The model under review builds one solid part; all positions refer to its coordinate system, in mm. A direction names the side the tool comes from. Give positions to 0.01 mm unless a question says otherwise; leave off trailing zeros. Order: outer loops, then holes, each group sorted by start corner. A loop starts at its lowest first (then second) coordinate and runs counter-clockwise, first axis right, second up. Notation, with made-up numbers: (32, -38.75) - (87, -38.75) arc R14 cw to (87, -17.75) - close; hole circle Ø3 at (-4.5, -16). An arc over 180 degrees is marked (long way). Write item = value, one per line. Start each with the question number.
1. We need section C-C, the plane z = -4.75. Give the boundary of the cut face in (x, y).
2. Wall thickness on probe 1 along X at (y, z) = (-35, -5.25); probe 2 along Y at (x, z) = (-35, 8.5); probe 3 along X at (y, z) = (-10, 11.5): over which ranges is each line inside the solid? List them lowest first.
3. Mouldability with a two-part tool opening along Y and no side actions: class faces 4 (the flat face through (-4, -22, 14)), 5 (the cylindrical face through (31.32, -43.472, 18.551)), 6 (the cylindrical face through (-31.836, -1.449, 18.472)), 7 (the cylindrical face through (37.21, -37.03, 5.21)) as pulls with the +Y half, pulls with the -Y half, needs draft (parallel to the pull), parting line crosses it, or undercut.
4. We need section B-B, the plane y = -10. Give the boundary of the cut face in (x, z).
5. Machinability: for faces 1 (the cylindrical face through (4.295, -43.472, 12.246)), 2 (the cylindrical face through (4.295, -1.528, 12.246)), 3 (the cylindrical face through (-10.202, -22.744, 19.404)), which of the approach directions +Z, -Z, +X, -X, +Y, -Y give a long, thin tool a straight path to every point of the face, cutting with its end or side? Answer none if there is none.
6. We need section A-A, the plane x = -35. Give the boundary of the cut face in (y, z).
7. For P1, Ø5, axis at x = -1, y = -10.5, coming from the +Z side; P2, Ø5, axis at x = -35, y = -35, coming from the -Z side, all flat-tipped, find the tip position at first contact; note any pin that passes through.
8. We need section D-D, the plane y = -27.5. Give the boundary of the cut face in (x, z).
from build123d import *

# Parameters (mm, degrees)
F1_DEPTH = 45
F2_R     = 7.62
F3_R     = 5.08
F5_D     = 6


with BuildPart() as f1:
    # F0 (on Front) → F1 (new body)
    with BuildSketch(Plane.XZ):
        Polygon((50, 20), (20, 20), (10, 20), (0, 10), (-10, 20), (-20, 20), (-50, 20), (-50, 0), (-50, -10), (50, -10), (50, 0), align=None)
    extrude(amount=F1_DEPTH)

    # F2
    f2_edges = [f1.edges().sort_by_distance(p)[0] for p in [
        (10, -22.5, 20),
        (-10, -22.5, 20),
    ]]
    fillet(f2_edges, radius=F2_R)

    # F3
    f3_edges = [f1.edges().sort_by_distance(p)[0] for p in [
        (-31.578154, -45, 20),
        (31.578154, -45, 20),
        (31.578154, 0, 20),
        (-31.578154, 0, 20),
    ]]
    fillet(f3_edges, radius=F3_R)

    # F5 (through all)
    with Locations(Plane(origin=(0, 0, -10), x_dir=(1, 0, 0), z_dir=(0, 0, -1))):
        with Locations((35, 10), (35, 35), (-35, 35), (-35, 10)):
            Hole(F5_D / 2)


solid = f1.part
Model answer:
q1.outline = (-50, -45) - (50, -45) - (50, 0) - (-50, 0) - close; hole circle Ø6 at (-35, -35); hole circle Ø6 at (-35, -10); hole circle Ø6 at (35, -35); hole circle Ø6 at (35, -10)
q2.probe_1 = -50 to -38, -32 to 32, 38 to 50
q2.probe_2 = -45 to -38, -32 to -13, -7 to 0
q2.probe_3 = -50 to -38, -32 to -1.5, 1.5 to 32, 38 to 50
q3.face_4 = needs draft
q3.face_5 = pulls with the -Y half
q3.face_6 = pulls with the +Y half
q3.face_7 = undercut
q4.outline = (-50, -10) - (-38, -10) - (-38, 20) - (-50, 20) - close; (-32, -10) - (32, -10) - (32, 20) - (13.16, 20) arc R7.62 ccw to (7.77, 17.77) - (0, 10) - (-7.77, 17.77) arc R7.62 ccw to (-13.16, 20) - (-32, 20) - close; (38, -10) - (50, -10) - (50, 20) - (38, 20) - close
q5.face_1 = +Z, -Y
q5.face_2 = +Z, +Y
q5.face_3 = +Z, +Y, -Y
q6.outline = (-45, -10) - (-38, -10) - (-38, 20) - (-39.92, 20) arc R5.08 ccw to (-45, 14.92) - close; (-32, -10) - (-13, -10) - (-13, 20) - (-32, 20) - close; (-7, -10) - (0, -10) - (0, 14.92) arc R5.08 ccw to (-5.08, 20) - (-7, 20) - close
q7.P1 = 13.5
q7.P2 = through
q8.outline = (-50, -10) - (50, -10) - (50, 20) - (13.16, 20) arc R7.62 ccw to (7.77, 17.77) - (0, 10) - (-7.77, 17.77) arc R7.62 ccw to (-13.16, 20) - (-50, 20) - close
